For this review, use the dimensioned drawing (mm, ordinates from the lowest corner) and the shaded views. Round coordinates to 2 decimals unless told otherwise and drop trailing zeros. Write each loop counter-clockwise with the first axis right and the second up, starting at its lowest first coordinate (ties: lowest second). Pieces come first, ordered by that corner, then holes. Notation, with made-up numbers: (-0.75, -37.5) -> (3.25, -37.5) arc R28 ccw to (3.25, -17.5) -> close; hole circle Ø7 at (-25, -35.5). An arc over 180 degrees is marked (long way). Answer in a Markdown table with one row per item. Add a question column.
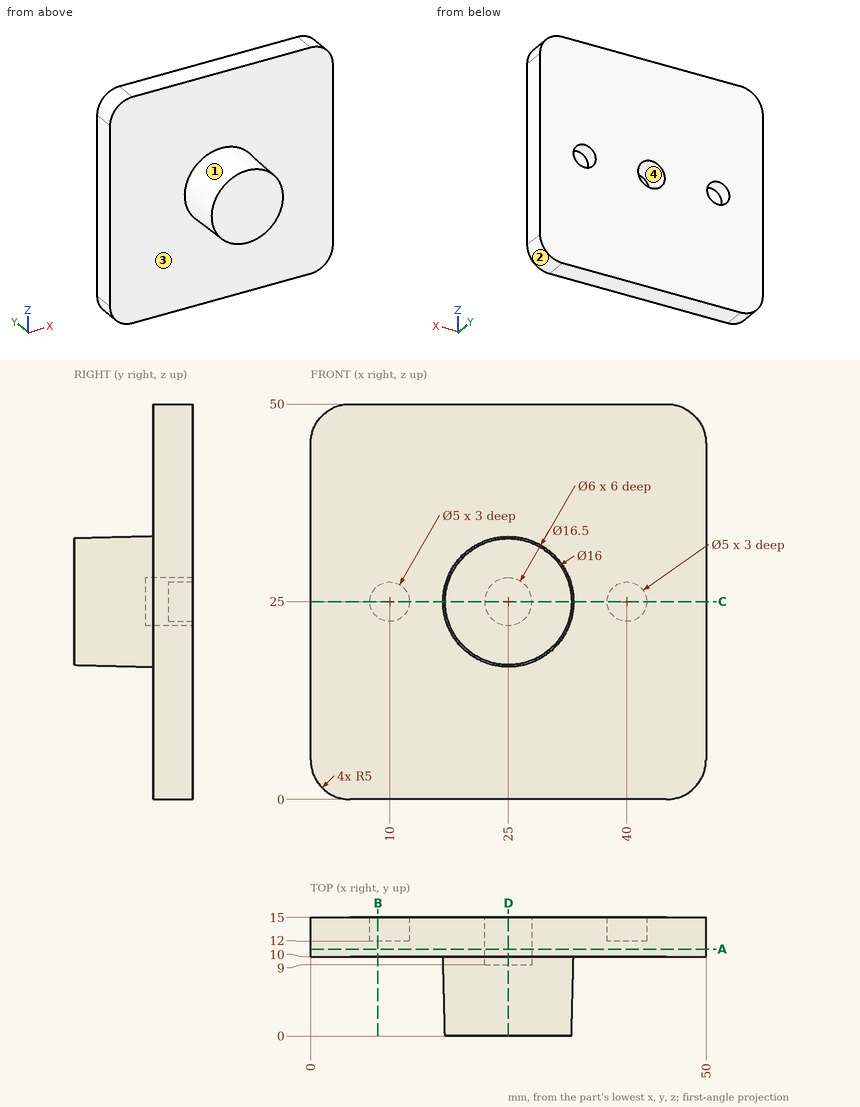
1. For L1, parallel to X at y = 12.7, z = 25; L2, parallel to Z at x = 10, y = 13.35; L3, parallel to X at y = 11.65, z = 25, list the stretches that pass through material, from the lowest coordinate up. Write a range as [from, to].
2. We need section C-C (z = 25). Write out the cut boundary in (x, y).
3. We need section B-B (x = 8.5). Write out the cut boundary in (y, z), plus the area to 3 significant figures.
4. We need section D-D (x = 25). Write out the cut boundary in (y, z).
5. We need section A-A (y = 11). Write out the cut boundary in (x, z), plus the area to 3 significant figures.
6. Clearance check with flat-ended pins moving along their axes: pin 1 Ø2 at (y, z) = (10, 31) entering from -X; pin 2 Ø1.5 at (x, z) = (10.5, 24.5) entering from +Y; pin 3 Ø1.5 at (x, z) = (26, 7) entering from -Y; pin 4 Ø1.5 at (y, z) = (7, 35) entering from -X. State where each tip first meets the part, or that it passes through.
7. The part is to be moulded in two halves that separate along X. For the marked faces 1, 2, 3 and 4, say which applies: pulls with the +X half, pulls with the -X half, needs draft (parallel to the pull), parting line crosses it, or undercut.
Response:
| question | item | result |
|---|---|---|
| 1 | L1 | [0, 7.5], [12.5, 22], [28, 37.5], [42.5, 50] |
| 1 | L2 | [0, 22.5], [27.5, 50] |
| 1 | L3 | [0, 22], [28, 50] |
| 2 | outline | (0, 10) -> (16.75, 10) -> (17, 0) -> (33, 0) -> (33.25, 10) -> (50, 10) -> (50, 15) -> (42.5, 15) -> (42.5, 12) -> (37.5, 12) -> (37.5, 15) -> (28, 15) -> (28, 9) -> (22, 9) -> (22, 15) -> (12.5, 15) -> (12.5, 12) -> (7.5, 12) -> (7.5, 15) -> (0, 15) -> close |
| 3 | outline | (10, 0) -> (15, 0) -> (15, 23) -> (12, 23) -> (12, 27) -> (15, 27) -> (15, 50) -> (10, 50) -> close |
| 3 | area | 238 mm2 |
| 4 | outline | (0, 17) -> (10, 16.75) -> (10, 0) -> (15, 0) -> (15, 22) -> (9, 22) -> (9, 28) -> (15, 28) -> (15, 50) -> (10, 50) -> (10, 33.25) -> (0, 33) -> close |
| 5 | outline | (0, 5) arc R5 ccw to (5, 0) -> (45, 0) arc R5 ccw to (50, 5) -> (50, 45) arc R5 ccw to (45, 50) -> (5, 50) arc R5 ccw to (0, 45) -> close; hole circle Ø6 at (25, 25) |
| 5 | area | 2,450 mm2 |
| 6 | pin 1 | x = 0 |
| 6 | pin 2 | y = 12 |
| 6 | pin 3 | y = 10 |
| 6 | pin 4 | through |
| 7 | face 1 | parting line crosses it |
| 7 | face 2 | pulls with the +X half |
| 7 | face 3 | needs draft |
| 7 | face 4 | undercut |
